Input: part model. Units: mm. Frame: model coordinates. Face numbers are marked on the shaded views. A direction names the side the tool comes from. Coordinates: 2 decimals unless noted, no trailing zeros. Loops run counter-clockwise (first coordinate to the right, second up) from the corner with the lowest first, then second, coordinate; pieces in that order, holes last. Notation, with made-up numbers: M -8.75,86.5 L 28.25,86.5 A13 ccw 28.25,98.5 Z; hole C 12,61.25 d7. An arc over 180 degrees is marked long. Use a Markdown table: item, result. Add a question column.
1. Pin query (flat end, axial travel): pin 1 (5 mm diameter, centred on x = 13.5, y = -7.5, fed in from -Z); pin 2 (1 mm diameter, centred on x = 7, z = -16, fed in from -Y); pin 3 (3 mm diameter, centred on y = -24, z = -20, fed in from +X). Return the tip coordinate at first contact, or that it passes through.
2. Section D-D on y = -48.5. Output: boundary loops of the cut face in (x, z).
3. Set-up query: the marked faces 1 and 2. Return all of +Z, -Z, +X, -X, +Y, -Y with unobstructed straight access to the full face (end or side cutting, diameter ignored); none if empty.
4. Line query: L1, parallel to Y at x = 11, z = 19; L2, parallel to Z at x = -26, y = -5; L3, parallel to X at y = -44, z = -0.5. Output: solid intervals per line, ascending. Write a range as [from, to].
5. Draft query along X for the marked faces 3, 4, 5 and 6. Return one class per face: +X half, -X half, draft (parallel to the pull), parting line (faces both ways), or undercut.
6. Section C-C on z = -13. Output: boundary loops of the cut face in (x, y).
7. Section A-A on x = 26. Output: boundary loops of the cut face in (y, z).
8. Section B-B on y = -8. Output: boundary loops of the cut face in (x, z), then the cut area to 3 significant figures.
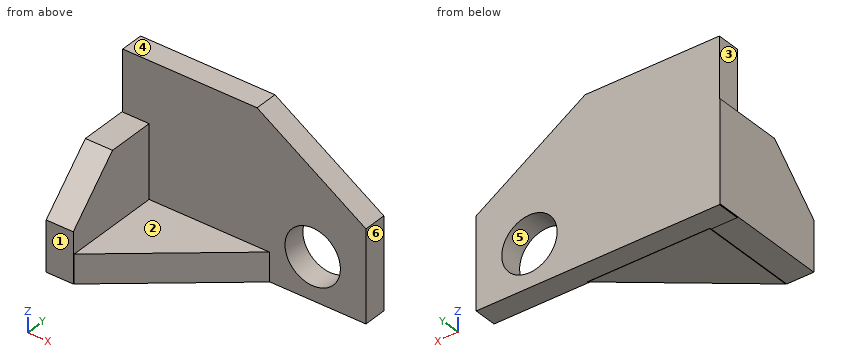
```python
from build123d import *

# Parameters (mm, degrees)
F0_R      = 12.5067254218
F1_DEPTH  = 10.414
F2_W      = 12.2419670224
F2_H      = 45.4701641575
F3_DEPTH  = 54.61
F4_SIZE   = 22.86
F6_DEPTH  = 30.734
F8_DEPTH  = 17.78
F9_W      = 56.2547529116
F9_H      = 22.1521309577
F10_DEPTH = 10.414


# Not quite as in the source:
# - a feature names something its author has since deleted; it is built from what else it names


with BuildPart() as f1:
    # F0 (on Front) → F1 (new body)
    with BuildSketch(Plane.XZ):
        Polygon((5.0146179641, 42.2928149286), (-55.6240000051, 42.2928149286), (-55.6240000051, -30.6337999585), (54.1666180116, -30.6337999585), (54.1666180116, 10.5042919132), align=None)
        with Locations((30.1248802542, -11.6675363407)):
            Circle(F0_R, mode=Mode.SUBTRACT)
    extrude(amount=F1_DEPTH)

    # F2 (on Front) → F3 (join)
    with BuildSketch(Plane.XZ):
        with Locations((-49.8422943056, -7.7240983956)):
            Rectangle(F2_W, F2_H)
    extrude(amount=F3_DEPTH)

    # F4
    f4_edges = [f1.edges().sort_by_distance(p)[0] for p in [
        (-49.842294, -54.61, 15.010984),
    ]]
    chamfer(f4_edges, length=F4_SIZE)

    # F5 (on Top) → F6 (join)
    with BuildSketch(Plane.XY):
        Polygon((11.3675408065, -9.7644263878), (-43.7213107944, -9.7644263878), (-43.7213107944, -54.0686920285), align=None)
    extrude(amount=-F6_DEPTH)

    # F7 (on Top) → F8 (cut)
    with BuildSketch(Plane.XY):
        Polygon((11.3675408065, -10.3473765776), (-43.7213107944, -10.3473765776), (-43.7213107944, -55.2345886827), align=None)
    extrude(amount=-F8_DEPTH, mode=Mode.SUBTRACT)

    # F9 (on Front) → F10 (join)
    with BuildSketch(Plane.XZ):
        with Locations((-15.5939343385, -6.8496719468)):
            Rectangle(F9_W, F9_H)
    extrude(amount=F10_DEPTH)


solid = f1.part
```
Answers below:
| question | item | result |
|---|---|---|
| 1 | pin 1 | stops at z = -30.63 |
| 1 | pin 2 | stops at y = -10.41 |
| 1 | pin 3 | stops at x = -4.47 |
| 2 | outline | M -55.96,-30.46 L -43.72,-30.46 L -43.72,-30.73 L -36.8,-30.73 L -36.8,-17.78 L -43.72,-17.78 L -43.72,-1.74 L -55.96,-1.74 Z |
| 3 | face 1 | +Z, -Z, +X, -X, -Y |
| 3 | face 2 | +Z, +X, -Y |
| 4 | L1 | y = [-10.41, 0] |
| 4 | L2 | z = [-30.63, 42.29] |
| 4 | L3 | x = [-55.96, -43.72] |
| 5 | face 3 | -X half |
| 5 | face 4 | draft |
| 5 | face 5 | undercut |
| 5 | face 6 | +X half |
| 6 | outline | M -55.96,-54.61 L -43.72,-54.61 L -43.72,-10.41 L 17.69,-10.41 L 17.69,0 L -55.96,0 Z; M 42.56,-10.41 L 54.17,-10.41 L 54.17,0 L 42.56,0 Z |
| 7 | outline | M -10.41,-30.63 L 0,-30.63 L 0,-23.47 L -10.41,-23.47 Z; M -10.41,0.14 L 0,0.14 L 0,28.72 L -10.41,28.72 Z |
| 8 | outline | M -55.96,-30.46 L -55.62,-30.46 L -55.62,-30.63 L 54.17,-30.63 L 54.17,10.5 L 5.01,42.29 L -55.62,42.29 L -55.62,15.01 L -55.96,15.01 Z; hole C 30.12,-11.67 d25.01 |
| 8 | area | 6,750 mm² |
